Here's how the part is built. I have some questions about the finished solid (model axes, mm). A direction names the side the tool comes from. Give positions to 0.01 mm unless a question says otherwise; leave off trailing zeros. Loops run counter-clockwise (first coordinate to the right, second up) from the corner with the lowest first, then second, coordinate; pieces in that order, holes last.
Q1. We'd pull the mould along Z, two halves only. Please class faces 1 (the face through (5, 0, 84)), 2 (the face through (5, 35, 42)), 3 (the face through (5.5, 2.3, 39)): +Z half, -Z half, draft (parallel to the pull), parting line (faces both ways), or undercut.
Q2. Will these pins go through, and if not, where does the flat tip stop? P1, Ø3, axis at x = 3.5, z = 68, coming from the -Y side (3 decimals); P2, Ø10, axis at y = -15, z = 7.5, coming from the -X side; P3, Ø7, axis at y = -15, z = 75.5, coming from the -X side; P4, Ø7.5, axis at y = 25, z = 42, coming from the +X side.
Q3. If we section it at A-A (z = 7.5): Please give me the cut outline in (x, y), plus the area to 3 significant figures.
Q4. I need wall thicknesses on line 1 (Z direction, x = 5, y = 0); line 2 (Y direction, x = 2.4, z = 7.5); line 3 (Y direction, x = 5.8, z = 7.5). Which ranges of each line are inside material? Lowest first, please.
Q5. For faces 4 (the face through (3.35, 0.09, 14.85)), 5 (the face through (8.32, -13.14, 40.15)), 6 (the face through (5, 22, 76)), 7 (the face through (4.2, -18, 8)), which set-ups out of +Z, -Z, +X, -X, +Y, -Y let a thin tool reach every point of the face, with its end or its side?
Q6. If we section it at B-B (x = 2.75): Give the number of separate pieces and of enclosed holes in the cut face, plus the area to 3 significant figures.
from build123d import *

# Parameters (mm, degrees)
CYLINDER014005932_R                                                    = 2.65
CYLINDER014005932_DEPTH                                                = 10
CYLINDER014005933_R                                                    = 2.65
CYLINDER014005933_DEPTH                                                = 10
CYLINDER014005934_R                                                    = 2.65
CYLINDER014005934_DEPTH                                                = 10
CYLINDER014005935_R                                                    = 4.3
CYLINDER014005935_DEPTH                                                = 4.2
CYLINDER014005936_R                                                    = 4.3
CYLINDER014005936_DEPTH                                                = 4.2
CYLINDER014005937_R                                                    = 4.3
CYLINDER014005937_DEPTH                                                = 4.2
CYLINDER014005938_R                                                    = 4.3
CYLINDER014005938_DEPTH                                                = 4.2
CYLINDER014005939_R                                                    = 2.65
CYLINDER014005939_DEPTH                                                = 10
CYLINDER014005940_R                                                    = 2.65
CYLINDER014005940_DEPTH                                                = 10
CYLINDER014005941_R                                                    = 4.3
CYLINDER014005941_DEPTH                                                = 4.2
CYLINDER014005942_R                                                    = 4.3
CYLINDER014005942_DEPTH                                                = 4.2
CYLINDER014005943_R                                                    = 3.15
CYLINDER014005943_DEPTH                                                = 10
PRISM010_DEPTH                                                         = 4.5
PRISM018_DEPTH                                                         = 3.4
CYLINDER014005962027_R                                                 = 2.15
CYLINDER014005962027_DEPTH                                             = 16
FUSION001089102007007003008034028016007006009018009018_PLACEMENT_ANGLE = 90
CYLINDER014005931_R                                                    = 2.65
CYLINDER014005931_DEPTH                                                = 10
BOX021002_W                                                            = 10
BOX021002_H                                                            = 44
BOX021002_DEPTH                                                        = 84
CYLINDER014005928_R                                                    = 35
CYLINDER014005928_DEPTH                                                = 10
CUT009003003009003003003007003002_PLACEMENT_ANGLE                      = 90
CHAMFER017_SIZE                                                        = 1
CHAMFER017_PLACEMENT_ANGLE                                             = 90


with BuildPart() as obj1:
    # Cylinder014005932 → Cylinder014005932 (new body)
    with BuildSketch(Plane(origin=(0, 15, 7.5), x_dir=(0, 0, -1), z_dir=(1, 0, 0))):
        Circle(CYLINDER014005932_R)
    extrude(amount=CYLINDER014005932_DEPTH)


with BuildPart() as obj2:
    # Cylinder014005933 → Cylinder014005933 (new body)
    with BuildSketch(Plane(origin=(0, -15, 75.5), x_dir=(0, 0, -1), z_dir=(1, 0, 0))):
        Circle(CYLINDER014005933_R)
    extrude(amount=CYLINDER014005933_DEPTH)


with BuildPart() as obj3:
    # Cylinder014005934 → Cylinder014005934 (new body)
    with BuildSketch(Plane(origin=(0, 15, 75.5), x_dir=(0, 0, -1), z_dir=(1, 0, 0))):
        Circle(CYLINDER014005934_R)
    extrude(amount=CYLINDER014005934_DEPTH)


with BuildPart() as obj4:
    # Cylinder014005935 → Cylinder014005935 (new body)
    with BuildSketch(Plane(origin=(0, -15, 7.5), x_dir=(0, 0, -1), z_dir=(1, 0, 0))):
        Circle(CYLINDER014005935_R)
    extrude(amount=CYLINDER014005935_DEPTH)


with BuildPart() as obj5:
    # Cylinder014005936 → Cylinder014005936 (new body)
    with BuildSketch(Plane(origin=(0, 15, 7.5), x_dir=(0, 0, -1), z_dir=(1, 0, 0))):
        Circle(CYLINDER014005936_R)
    extrude(amount=CYLINDER014005936_DEPTH)


with BuildPart() as obj6:
    # Cylinder014005937 → Cylinder014005937 (new body)
    with BuildSketch(Plane(origin=(0, -15, 75.5), x_dir=(0, 0, -1), z_dir=(1, 0, 0))):
        Circle(CYLINDER014005937_R)
    extrude(amount=CYLINDER014005937_DEPTH)


with BuildPart() as obj7:
    # Cylinder014005938 → Cylinder014005938 (new body)
    with BuildSketch(Plane(origin=(0, 15, 75.5), x_dir=(0, 0, -1), z_dir=(1, 0, 0))):
        Circle(CYLINDER014005938_R)
    extrude(amount=CYLINDER014005938_DEPTH)


with BuildPart() as obj8:
    # Cylinder014005939 → Cylinder014005939 (new body)
    with BuildSketch(Plane(origin=(0, -25, 42), x_dir=(0, 0, -1), z_dir=(1, 0, 0))):
        Circle(CYLINDER014005939_R)
    extrude(amount=CYLINDER014005939_DEPTH)


with BuildPart() as obj9:
    # Cylinder014005940 → Cylinder014005940 (new body)
    with BuildSketch(Plane(origin=(0, 25, 42), x_dir=(0, 0, -1), z_dir=(1, 0, 0))):
        Circle(CYLINDER014005940_R)
    extrude(amount=CYLINDER014005940_DEPTH)


with BuildPart() as obj10:
    # Cylinder014005941 → Cylinder014005941 (new body)
    with BuildSketch(Plane(origin=(5.8, -25, 42), x_dir=(0, 0, -1), z_dir=(1, 0, 0))):
        Circle(CYLINDER014005941_R)
    extrude(amount=CYLINDER014005941_DEPTH)


with BuildPart() as obj11:
    # Cylinder014005942 → Cylinder014005942 (new body)
    with BuildSketch(Plane(origin=(5.8, 25, 42), x_dir=(0, 0, -1), z_dir=(1, 0, 0))):
        Circle(CYLINDER014005942_R)
    extrude(amount=CYLINDER014005942_DEPTH)


with BuildPart() as obj12:
    # Cylinder014005943 → Cylinder014005943 (new body)
    with BuildSketch(Plane(origin=(0, 0, 0), x_dir=(0, 0, -1), z_dir=(1, 0, 0))):
        Circle(CYLINDER014005943_R)
    extrude(amount=CYLINDER014005943_DEPTH)


with BuildPart() as fusion001089102007007003008034028016004:
    # Prism010 → Prism010 (new body)
    with BuildSketch(Plane(origin=(5.5, 0, 0), x_dir=(0, 0, -1), z_dir=(1, 0, 0))):
        Polygon((5.8, 0), (2.9, 5.022947), (-2.9, 5.022947), (-5.8, 0), (-2.9, -5.022947), (2.9, -5.022947), align=None)
    extrude(amount=PRISM010_DEPTH)

    # Fusion001089102007007003008034028016004: union obj12
    add(obj12.part)


with BuildPart() as fusion001089102007007003008034028016004_1:
    # Fusion001089102007007003008034028016004 placement: moved
    add(fusion001089102007007003008034028016004.part.moved(Location((0, 0, 41.5))))


with BuildPart() as m4x010:
    # prism018 → prism018 (new body)
    with BuildSketch(Plane(origin=(0, 0, 0), x_dir=(0, 1, 0), z_dir=(0, 0, 1))):
        Polygon((4.21, 0), (2.105, 3.645967), (-2.105, 3.645967), (-4.21, 0), (-2.105, -3.645967), (2.105, -3.645967), align=None)
    extrude(amount=PRISM018_DEPTH)


with BuildPart() as m4nut042:
    # Cylinder014005962027 → Cylinder014005962027 (new body)
    with BuildSketch(Plane.XY):
        Circle(CYLINDER014005962027_R)
    extrude(amount=CYLINDER014005962027_DEPTH)

    # Fusion001089102007007003008034028016007006009018009018: union M4X010
    add(m4x010.part)


with BuildPart() as m4nut042_1:
    # Fusion001089102007007003008034028016007006009018009018 placement: moved
    add(m4nut042.part.moved(Location((10, 0, 42))).rotate(Axis((10, 0, 42), (0, -1, 0)), FUSION001089102007007003008034028016007006009018009018_PLACEMENT_ANGLE))


with BuildPart() as m4nut043:
    # Fusion001089102007007003008034028016007006009018009019 base: copy of M4nut042
    add(m4nut042_1.part)


with BuildPart() as m4nut043_1:
    # Fusion001089102007007003008034028016007006009018009019 placement: moved
    add(m4nut043.part.moved(Location((0, 10, 0))))


with BuildPart() as m4nut044:
    # Fusion001089102007007003008034028016007006009018009020 base: copy of M4nut042
    add(m4nut042_1.part)


with BuildPart() as m4nut044_1:
    # Fusion001089102007007003008034028016007006009018009020 placement: moved
    add(m4nut044.part.moved(Location((0, -10, 0))))


with BuildPart() as m4nut046:
    # Fusion001089102007007003008034028016007006009018009022 base: copy of M4nut042
    add(m4nut042_1.part)


with BuildPart() as m4nut046_1:
    # Fusion001089102007007003008034028016007006009018009022 placement: moved
    add(m4nut046.part.moved(Location((0, 0, -25))))


with BuildPart() as m4nut045:
    # Fusion001089102007007003008034028016007006009018009021 base: copy of M4nut042
    add(m4nut042_1.part)


with BuildPart() as m4nut045_1:
    # Fusion001089102007007003008034028016007006009018009021 placement: moved
    add(m4nut045.part.moved(Location((0, 0, 25))))


with BuildPart() as fusion001089102007007003008034028016003:
    # Cylinder014005931 → Cylinder014005931 (new body)
    with BuildSketch(Plane(origin=(0, -15, 7.5), x_dir=(0, 0, -1), z_dir=(1, 0, 0))):
        Circle(CYLINDER014005931_R)
    extrude(amount=CYLINDER014005931_DEPTH)

    # Fusion001089102007007003008034028016003: union obj1, obj2, obj3, obj4, obj5, obj6, obj7, obj8, obj9, obj10, obj11, Fusion001089102007007003008034028016004, M4nut043, M4nut044, M4nut046, M4nut045
    add(obj1.part)
    add(obj2.part)
    add(obj3.part)
    add(obj4.part)
    add(obj5.part)
    add(obj6.part)
    add(obj7.part)
    add(obj8.part)
    add(obj9.part)
    add(obj10.part)
    add(obj11.part)
    add(fusion001089102007007003008034028016004_1.part)
    add(m4nut043_1.part)
    add(m4nut044_1.part)
    add(m4nut046_1.part)
    add(m4nut045_1.part)


with BuildPart() as krychle024:
    # Box021002 → Box021002 (new body)
    with BuildSketch(Plane(origin=(0, -22, 0), x_dir=(1, 0, 0), z_dir=(0, 0, 1))):
        with Locations((5, 22)):
            Rectangle(BOX021002_W, BOX021002_H)
    extrude(amount=BOX021002_DEPTH)


with BuildPart() as obj13:
    # Cylinder014005928 → Cylinder014005928 (new body)
    with BuildSketch(Plane(origin=(0, 0, 42), x_dir=(0, 0, -1), z_dir=(1, 0, 0))):
        Circle(CYLINDER014005928_R)
    extrude(amount=CYLINDER014005928_DEPTH)

    # Fusion001089102007007003008034028016002: union Krychle024
    add(krychle024.part)

    # Cut009003003009003003003007003002: cut Fusion001089102007007003008034028016003
    add(fusion001089102007007003008034028016003.part, mode=Mode.SUBTRACT)


with BuildPart() as obj13_1:
    # Cut009003003009003003003007003002 placement: moved
    add(obj13.part.rotate(Axis((0, 0, 0), (1, 0, 0)), CUT009003003009003003003007003002_PLACEMENT_ANGLE))

    # Chamfer017
    chamfer017_edges = [obj13_1.edges().sort_by_distance(p)[0] for p in [
        (0, -42, -35),
        (10, -42, -35),
        (10, -76.610658, -22),
        (5, -84, -22),
        (0, -76.610658, -22),
        (0, -84, 0),
        (5, -84, 22),
        (10, -84, 0),
        (10, -76.610658, 22),
        (0, -76.610658, 22),
        (10, -42, 35),
        (0, -42, 35),
        (10, -7.389342, -22),
        (0, -7.389342, -22),
        (5, 0, -22),
        (10, -7.389342, 22),
        (0, -7.389342, 22),
        (5, 0, 22),
        (0, 0, 0),
        (10, 0, 0),
    ]]
    chamfer(chamfer017_edges, length=CHAMFER017_SIZE)


with BuildPart() as obj13_2:
    # Chamfer017 placement: moved
    add(obj13_1.part.rotate(Axis((0, 0, 0), (-1, 0, 0)), CHAMFER017_PLACEMENT_ANGLE))


solid = obj13_2.part
Check sheet entries:
1. face 1: +Z half
1. face 2: parting line
1. face 3: undercut
2. P1: stops at y = -24.995
2. P2: stops at x = 0
2. P3: stops at x = 4.2
2. P4: stops at x = 5.8
3. outline: (0, -21) - (1, -22) - (9, -22) - (10, -21) - (10, -17.65) - (4.2, -17.65) - (4.2, -19.3) - (0, -19.3) - close; (0, -10.7) - (4.2, -10.7) - (4.2, -12.35) - (10, -12.35) - (10, 12.35) - (4.2, 12.35) - (4.2, 10.7) - (0, 10.7) - close; (0, 19.3) - (4.2, 19.3) - (4.2, 17.65) - (10, 17.65) - (10, 21) - (9, 22) - (1, 22) - (0, 21) - close
3. area: 304 mm2
4. line 1: z = 0 to 14.85, 19.15 to 38.35, 44.65 to 64.85, 69.15 to 84
4. line 2: y = -22 to -19.3, -10.7 to 10.7, 19.3 to 22
4. line 3: y = -22 to -17.65, -12.35 to 12.35, 17.65 to 22
5. face 4: +X, -X
5. face 5: +X
5. face 6: +Z, +X, -X, +Y
5. face 7: -X
6. separate pieces: 1
6. enclosed holes: 11
6. area: 4,310 mm2
